Part model, mm, in its own coordinate system. A direction names the side the tool comes from. Coordinates: 2 decimals unless noted, no trailing zeros. Loops run counter-clockwise (first coordinate to the right, second up) from the corner with the lowest first, then second, coordinate; pieces in that order, holes last. Notation, with made-up numbers: (84, 11.25) - (116, 11.25) arc R18 cw to (116, 25.25) - close; hole circle Ø5 at (65, -23). An arc over 180 degrees is marked (long way). Use a Markdown table: item, result. Add a question column.
1) Band-saw the part on D-D (x = 14). Give the cut face in (y, z), plus the area to 3 significant figures.
2) Drop flat-ended pins along their axis: P1, Ø4, axis at y = 50.57, z = 7.5, coming from the -X side; P2, Ø6, axis at x = 27.5, z = 9, coming from the +Y side; P3, Ø5.5, axis at y = 38.5, z = 8.5, coming from the -X side; P4, Ø4, axis at x = 28, z = 6.5, coming from the +Y side. Give the stop position or say it passes through.
3) Band-saw the part on C-C (z = 5.5). Give the number of separate pieces and of enclosed holes in the cut face, plus the area to 3 significant figures.
4) Pull direction X, two halves, no side cores. Call faces 1 (the face through (35.03, 54.04, 12.89)), 2 (the face through (2.6, -3, 12.9)), 3 (the face through (4.385, -2.958, 4.395)): +X half, -X half, draft (parallel to the pull), parting line (faces both ways), or undercut.
5) Band-saw the part on B-B (y = 31.5). Give the cut face in (x, z), plus the area to 3 significant figures.
6) Probe probe 1 along X at (y, z) = (47, 9.5); probe 2 along Y at (x, z) = (10.5, 10.25); probe 3 along Y at (x, z) = (35.8, 7.5). List the from-to ranges inside material, lowest first. Write a range as [from, to].
7) Tool access for faces 4 (the face through (31.57, 29.89, 0.6)), 5 (the face through (13, 0, 7)), 6 (the face through (33.958, 47.152, 6.741)), 7 (the face through (31.6, 29.89, 14.43)): list every direction of +Z, -Z, +X, -X, +Y, -Y with a clear straight run to the whole face (end or side of a thin tool).
8) Band-saw the part on A-A (x = 6). Give the cut face in (y, z), plus the area to 3 significant figures.
from build123d import *

# Parameters (mm, degrees)
EXTRUDE_1_DEPTH     = 15
SKETCH_3_R          = 3.5
CUT_EXTRUDE_1_DEPTH = 70.286826712
SKETCH_4_R          = 3.5
CUT_EXTRUDE_2_DEPTH = 67.277178243
FILLET_1_R          = 8
FILLET_4_R          = 2


with BuildPart() as part:
    # 草图1 → 凸台-拉伸1 (new body)
    with BuildSketch(Plane.XY):
        Polygon((0, 0), (0, -6), (22.857864376, -6), (37, 8.142135624), (37, 56.627416998), (31, 56.627416998), (31, 10.627416998), (20.372583002, 0), align=None)
    extrude(amount=EXTRUDE_1_DEPTH)

    # 草图3 → 切除-拉伸1 (cut, through all)
    with BuildSketch(Plane(origin=(0, 0, 0), x_dir=(1, 0, 0), z_dir=(0, 1, 0))):
        with Locations(Location((6, -7.5, 0), (0, 0, 180))):
            Circle(SKETCH_3_R)
    extrude(amount=-CUT_EXTRUDE_1_DEPTH, mode=Mode.SUBTRACT)

    # 草图4 → 切除-拉伸2 (cut, through all)
    with BuildSketch(Plane.ZY.offset(-31)):
        with Locations((7.5, 50.568542495)):
            Circle(SKETCH_4_R)
    extrude(amount=-CUT_EXTRUDE_2_DEPTH, mode=Mode.SUBTRACT)

    # 圆角1
    # the kernel refuses this fillet: 8 mm, written as the material it takes off along each edge
    with BuildSketch(Plane(origin=(0, 20, 15), x_dir=(0, 0, -1), z_dir=(0, -1, 0)), Plane(origin=(57, 56.627416998, 0), x_dir=(0, -1, 0), z_dir=(-1, 0, 0))) as fillet_1_piece_1:
        with BuildLine():
            CenterArc((FILLET_1_R, FILLET_1_R), FILLET_1_R, 180, 90)
            Line((0, FILLET_1_R), (0, 0))
            Line((0, 0), (FILLET_1_R, 0))
        make_face()
    extrude(amount=46, mode=Mode.SUBTRACT)
    with BuildSketch(Plane(origin=(0, 20, 0), x_dir=(0, 0, 1), z_dir=(0, -1, 0)), Plane(origin=(57, 56.627416998, 15), x_dir=(0, -1, 0), z_dir=(-1, 0, 0))) as fillet_1_piece_2:
        with BuildLine():
            CenterArc((FILLET_1_R, -FILLET_1_R), FILLET_1_R, 90, 90)
            Line((0, -FILLET_1_R), (0, 0))
            Line((0, 0), (FILLET_1_R, 0))
        make_face()
    extrude(amount=46, mode=Mode.SUBTRACT)

    # 圆角4
    # the kernel refuses this fillet: 2 mm, written as the material it takes off along each edge
    with BuildSketch(Plane(origin=(31, 48.627416998, 15), x_dir=(0, 0, -1), z_dir=(0, -1, 0))) as fillet_4_piece_1_section:
        with BuildLine():
            CenterArc((FILLET_4_R, FILLET_4_R), FILLET_4_R, 180, 90)
            Line((0, FILLET_4_R), (0, 0))
            Line((0, 0), (FILLET_4_R, 0))
        make_face()
    fillet_4_piece_1 = extrude(amount=43, mode=Mode.PRIVATE)
    fillet_4_piece_1 = split(fillet_4_piece_1, bisect_by=Plane(origin=(40.835879215, 20.463296213, 14.544284738), z_dir=(-0.7071067811865489, 0.7071067811865461, 0)), keep=Keep.TOP, mode=Mode.PRIVATE)
    add(fillet_4_piece_1, mode=Mode.SUBTRACT)
    with BuildSketch(Plane(origin=(31, 48.627416998, 0), x_dir=(1, 0, 0), z_dir=(0, -1, 0))) as fillet_4_piece_2_section:
        with BuildLine():
            CenterArc((FILLET_4_R, FILLET_4_R), FILLET_4_R, 180, 90)
            Line((0, FILLET_4_R), (0, 0))
            Line((0, 0), (FILLET_4_R, 0))
        make_face()
    fillet_4_piece_2 = extrude(amount=43, mode=Mode.PRIVATE)
    fillet_4_piece_2 = split(fillet_4_piece_2, bisect_by=Plane(origin=(40.835879215, 20.463296213, 0.455715262), z_dir=(-0.7071067811865489, 0.7071067811865461, 0)), keep=Keep.TOP, mode=Mode.PRIVATE)
    add(fillet_4_piece_2, mode=Mode.SUBTRACT)
    with BuildSketch(Plane(origin=(31, 48.627416998, 7), x_dir=(0, 0.8458227796369704, -0.5334639870199197), z_dir=(0, -0.5334639870199197, -0.8458227796369704))) as fillet_4_piece_3:
        with BuildLine():
            CenterArc((8 - FILLET_4_R, FILLET_4_R), FILLET_4_R, 270, 90)
            Line((8, FILLET_4_R), (8, 0))
            Line((8, 0), (8 - FILLET_4_R, 0))
        make_face()
    revolve(axis=Axis((31, 48.627416998, 7), (1, 0, 0)), revolution_arc=122.239802646, mode=Mode.SUBTRACT)
    with BuildSketch(Plane(origin=(31, 48.627416998, 8), x_dir=(0, 0, -1), z_dir=(0, -1, 0))) as fillet_4_piece_4:
        with BuildLine():
            CenterArc((8 - FILLET_4_R, FILLET_4_R), FILLET_4_R, 270, 90)
            Line((8, FILLET_4_R), (8, 0))
            Line((8, 0), (8 - FILLET_4_R, 0))
        make_face()
    revolve(axis=Axis((31, 48.627416998, 8), (1, 0, 0)), revolution_arc=122.239802646, mode=Mode.SUBTRACT)


solid = part.part
Answer block:
| question | item | result |
|---|---|---|
| 1 | outline | (-6, 0) - (0, 0) - (0, 15) - (-6, 15) - close |
| 1 | area | 90.0 mm2 |
| 2 | P1 | through |
| 2 | P2 | y = 10.13 |
| 2 | P3 | x = 31 |
| 2 | P4 | y = 9.63 |
| 3 | separate pieces | 3 |
| 3 | enclosed holes | 0 |
| 3 | area | 444 mm2 |
| 4 | face 1 | draft |
| 4 | face 2 | -X half |
| 4 | face 3 | undercut |
| 5 | outline | (31, 2) arc R2 ccw to (33, 0) - (37, 0) - (37, 15) - (33, 15) arc R2 ccw to (31, 13) - close |
| 5 | area | 88.3 mm2 |
| 6 | probe 1 | [31, 37] |
| 6 | probe 2 | [-6, 0] |
| 6 | probe 3 | [6.94, 47.07], [54.07, 56.61] |
| 7 | face 4 | -Z, -X, +Y |
| 7 | face 5 | +Z, -Z, -X, +Y |
| 7 | face 6 | +X, -X |
| 7 | face 7 | +Z, -X, +Y |
| 8 | outline | (-6, 0.25) - (0, 0.25) - (0, 4) - (-6, 4) - close; (-6, 11) - (0, 11) - (0, 14.75) - (-6, 14.75) - close |
| 8 | area | 45.0 mm2 |
